Geometry check sheet. Reference: the model listing, model coordinates, mm. Face numbers are marked on the shaded views. A direction names the side the tool comes from. Round coordinates to 2 decimals unless told otherwise and drop trailing zeros. Write each loop counter-clockwise with the first axis right and the second up, starting at its lowest first coordinate (ties: lowest second). Pieces come first, ordered by that corner, then holes. Notation, with made-up numbers: M 36.25,8 L 41.25,8 A10 cw 41.25,25 Z; hole C -11,-18.5 d8. An arc over 180 degrees is marked long. Answer as CSV lines item,"result". Start each with the question number.
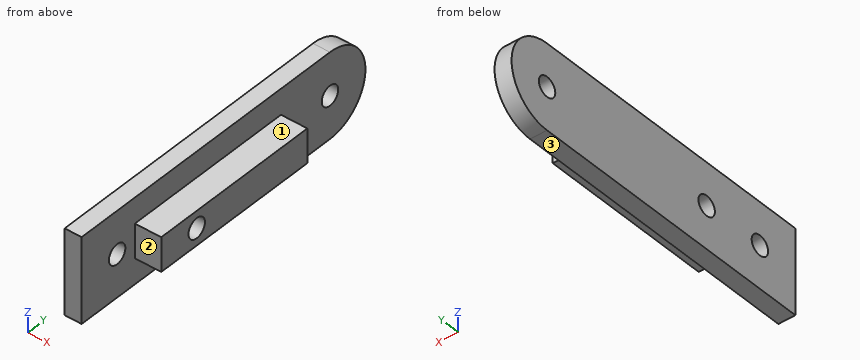
```python
from build123d import *

# Parameters (mm, degrees)
BOSS_EXTRUDE1_DEPTH     = 2.54
SKETCH2_W               = 5.08
SKETCH2_H               = 26.152706233
BOSS_EXTRUDE2_DEPTH     = 3.937
CUT_EXTRUDE1_DEPTH      = 46.366028358
CUT_EXTRUDE1_DEPTH_BACK = 46.366028358
SKETCH3_R               = 1.4732
F_4_CLEARANCE_HOLE1_D   = 2.9464


with BuildPart() as part:
    # Sketch1 → Boss-Extrude1 (new body)
    with BuildSketch(Plane(origin=(0, 0, 0), x_dir=(0, 0, -1), z_dir=(1, 0, 0))):
        with BuildLine():
            Line((6.35, -44.45), (6.35, 0))
            ThreePointArc((6.35, 0), (0, 6.35), (-6.35, 0))
            Line((-6.35, 0), (-6.35, -44.45))
            Line((-6.35, -44.45), (6.35, -44.45))
        make_face()
    extrude(amount=BOSS_EXTRUDE1_DEPTH)

    # Sketch2 → Boss-Extrude2 (add)
    with BuildSketch(Plane(origin=(2.54, 0, 0), x_dir=(0, 0, -1), z_dir=(1, 0, 0))):
        with Locations((0, -21.848646884)):
            Rectangle(SKETCH2_W, SKETCH2_H)
    extrude(amount=BOSS_EXTRUDE2_DEPTH)

    # Sketch3 → Cut-Extrude1 (cut, two sides: drawn at the far end of the back side and taken through both)
    with BuildSketch(Plane.ZY.offset(-CUT_EXTRUDE1_DEPTH_BACK)):
        with Locations(Location((0, 0, 0), (0, 0, 180))):
            Circle(SKETCH3_R)
    extrude(amount=CUT_EXTRUDE1_DEPTH + CUT_EXTRUDE1_DEPTH_BACK, mode=Mode.SUBTRACT)

    # #4 Clearance Hole1 (through all)
    with Locations(Plane.ZY):
        with Locations((0, -28.575), (0, -38.1)):
            Hole(F_4_CLEARANCE_HOLE1_D / 2)


solid = part.part
```
1) Scan lines: line 1 (Y direction, x = 2, z = 0); line 2 (Y direction, x = 0.75, z = -0.5); line 3 (X direction, y = -36, z = 1). Record each from-to range of solid material in increasing order. Write a range as from..to.
2) Section check B-B, the plane z = 0. Record the cut outline in (x, y) (3 decimals), plus the area to 3 significant figures.
3) Access from +Z, -Z, +X, -X, +Y, -Y to the whole of each face (thin tool, end or side, straight path). Record for the marked faces 1, 2 and 3.
4) Go/stop test with flat-tipped pins: pin 1 (2.5 mm diameter, centred on y = 0, z = 0, fed in from -X); pin 2 (1.5 mm diameter, centred on x = 1.5, z = -1.5, fed in from +Y); pin 3 (5 mm diameter, centred on y = 0, z = -5, fed in from +X); pin 4 (3 mm diameter, centred on x = 5, z = 1, fed in from +Y). Record where each tip stops, or that it passes through.
5) Section check C-C, the plane x = 2. Record the cut outline in (y, z) (3 decimals), plus the area to 3 significant figures.
6) Section check A-A, the plane y = -38.1. Record the cut outline in (x, z).
7) Section check D-D, the plane y = -32. Record the cut outline in (x, z), plus the area to 3 significant figures.
Results:
1,line 1,"y = -44.45..-39.57, -36.63..-30.05, -27.1..-1.47, 1.47..6.35"
1,line 2,"y = -44.45..-39.49, -36.71..-29.96, -27.19..-1.39, 1.39..6.33"
1,line 3,"x = 0..2.54"
2,outline,"M 0,-44.45 L 2.54,-44.45 L 2.54,-39.573 L 0,-39.573 Z; M 0,-36.627 L 2.54,-36.627 L 2.54,-34.925 L 6.477,-34.925 L 6.477,-30.048 L 0,-30.048 Z; M 0,-27.102 L 6.477,-27.102 L 6.477,-8.772 L 2.54,-8.772 L 2.54,-1.473 L 0,-1.473 Z; M 0,1.473 L 2.54,1.473 L 2.54,6.35 L 0,6.35 Z"
2,area,"198 mm^2"
3,face 1,"+Z, +X, +Y, -Y"
3,face 2,"+Z, -Z, +X, -Y"
3,face 3,"-Z, +X, -X, +Y, -Y"
4,pin 1,"passes through"
4,pin 2,"stops at y = 6.31"
4,pin 3,"stops at x = 2.54"
4,pin 4,"stops at y = -8.77"
5,outline,"M -44.45,-6.35 L 0,-6.35 A6.35 ccw 0,6.35 L -44.45,6.35 Z; hole C -38.1,0 d2.946; hole C -28.575,0 d2.946; hole C 0,0 d2.946"
5,area,"607 mm^2"
6,outline,"M 0,-6.35 L 2.54,-6.35 L 2.54,-1.47 L 0,-1.47 Z; M 0,1.47 L 2.54,1.47 L 2.54,6.35 L 0,6.35 Z"
7,outline,"M 0,-6.35 L 2.54,-6.35 L 2.54,-2.54 L 6.48,-2.54 L 6.48,2.54 L 2.54,2.54 L 2.54,6.35 L 0,6.35 Z"
7,area,"52.3 mm^2"
